Can you work these out from the drawing? Everything is in mm from the part's minimum corner. A direction names the side the tool comes from. Coordinates: 2 decimals unless noted, no trailing zeros. Loops run counter-clockwise (first coordinate to the right, second up) from the corner with the lowest first, then second, coordinate; pieces in that order, holes last.
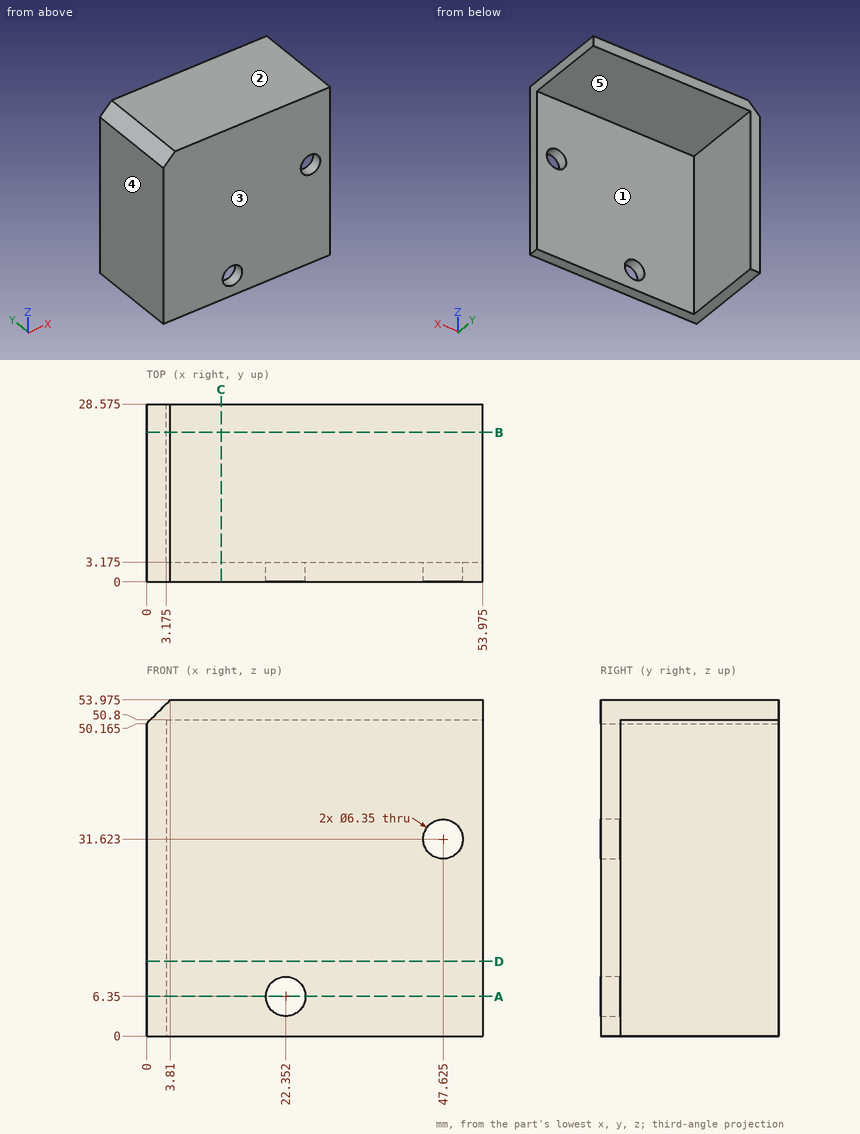
1) Imagine slicing it at D-D on z = 12. List the corners of the cut face in (x, y) for me (3 decimals), plus the area to 3 significant figures.
2) Imagine slicing it at C-C on x = 12. List the corners of the cut face in (y, z) for me (3 decimals).
3) If I drill on L1, parallel to X at y = 0.85, z = 6.35 (3 decimals); L2, parallel to Z at x = 14.5, y = 7 (3 decimals); L3, parallel to Y at x = 17.5, z = 18 (3 decimals), over which ranges is the centre line in solid material (lowest first)?
4) Imagine slicing it at B-B on y = 24. List the corners of the cut face in (x, z) for me (3 decimals).
5) For the marked faces 4 and 5, which set-ups out of +Z, -Z, +X, -X, +Y, -Y let a thin tool reach every point of the face, with its end or its side?
6) We'd pull the mould along Y, two halves only. Please class the marked faces 1, 2 and 3: released by +Y, released by -Y, zero draft, split by the parting line, or undercut.
7) Imagine slicing it at A-A on z = 6.35. List the corners of the cut face in (x, y) for me (3 decimals), plus the area to 3 significant figures.
8) Will these pins go through, and if not, where does the flat tip stop? pin 1 (8 mm diameter, centred on x = 35, z = 28.5, fed in from -Y); pin 2 (12.5 mm diameter, centred on y = 20.5, z = 34, fed in from +X) (3 decimals); pin 3 (1 mm diameter, centred on x = 25, z = 45, fed in from +Y) (3 decimals).
Solved:
1. outline: (0, 0) - (53.975, 0) - (53.975, 3.175) - (3.175, 3.175) - (3.175, 28.575) - (0, 28.575) - close
1. area: 252 mm2
2. outline: (0, 0) - (3.175, 0) - (3.175, 50.8) - (28.575, 50.8) - (28.575, 53.975) - (0, 53.975) - close
3. L1: x = 0 to 19.177, 25.527 to 53.975
3. L2: z = 50.8 to 53.975
3. L3: y = 0 to 3.175
4. outline: (0, 0) - (3.175, 0) - (3.175, 50.8) - (53.975, 50.8) - (53.975, 53.975) - (3.81, 53.975) - (0, 50.165) - close
5. face 4: +Z, -Z, -X, +Y, -Y
5. face 5: -Z, +X, +Y
6. face 1: released by +Y
6. face 2: zero draft
6. face 3: released by -Y
7. outline: (0, 0) - (19.177, 0) - (19.177, 3.175) - (3.175, 3.175) - (3.175, 28.575) - (0, 28.575) - close; (25.527, 0) - (53.975, 0) - (53.975, 3.175) - (25.527, 3.175) - close
7. area: 232 mm2
8. pin 1: stops at y = 0
8. pin 2: stops at x = 3.175
8. pin 3: stops at y = 3.175
